from build123d import *

# Parameters (mm, degrees)
F1_DEPTH = 25.4
F2_R     = 3.175
F3_W     = 25.4
F3_H     = 6.35
F4_DEPTH = 53.976


with BuildPart() as f1:
    # F0 (on Front) → F1 (new body)
    with BuildSketch(Plane.XZ):
        with BuildLine():
            Line((-85.615239, 25.710709), (-159.144036, 1.439067))
            ThreePointArc((-159.144036, 1.439067), (-162.299532, -0.870485), (-163.503562, -4.590901))
            Line((-163.503562, -4.590901), (-163.503562, -26.984162))
            Line((-163.503562, -26.984162), (-81.740962, -26.984162))
            ThreePointArc((-81.740962, -26.984162), (-79.88109, -22.494034), (-75.390962, -20.634162))
            Line((-75.390962, -20.634162), (0, -20.634162))
            Line((0, -20.634162), (75.390962, -20.634162))
            ThreePointArc((75.390962, -20.634162), (79.88109, -22.494034), (81.740962, -26.984162))
            Line((81.740962, -26.984162), (163.503562, -26.984162))
            Line((163.503562, -26.984162), (163.503562, -4.590901))
            ThreePointArc((163.503562, -4.590901), (162.299532, -0.870485), (159.144036, 1.439067))
            Line((159.144036, 1.439067), (85.615239, 25.710709))
            ThreePointArc((85.615239, 25.710709), (81.685416, 26.668764), (77.65334, 26.990838))
            Line((77.65334, 26.990838), (0, 26.990838))
            Line((0, 26.990838), (-77.65334, 26.990838))
            ThreePointArc((-77.65334, 26.990838), (-81.685416, 26.668764), (-85.615239, 25.710709))
        make_face()
    extrude(amount=F1_DEPTH)

    # F2
    f2_edges = [f1.edges().sort_by_distance(p)[0] for p in [
        (-163.503562, -25.4, -15.787532),
        (-162.299532, -25.4, -0.870485),
        (-122.379638, -25.4, 13.574888),
        (122.379638, 0, 13.574888),
        (-163.503562, -12.7, -26.984162),
        (163.503562, -12.7, -26.984162),
    ]]
    fillet(f2_edges, radius=F2_R)

    # F3 (on face) → F4 (cut, through all)
    with BuildSketch(Plane.XY.offset(26.990838)):
        with Locations((0, -12.7)):
            Rectangle(F3_W, F3_H)
    extrude(amount=-F4_DEPTH, mode=Mode.SUBTRACT)


solid = f1.part
Design review of the part built by this model. Coordinates are the model's own, in mm. A direction names the side the tool comes from. Coordinates: 2 decimals unless noted, no trailing zeros. Order: outer loops, then holes, each group sorted by start corner. A loop starts at its lowest first (then second) coordinate and runs counter-clockwise, first axis right, second up.
Item 1: Take a section at B-B, the plane y = -12.75. Write out the cut boundary in (x, z) (3 decimals), then the cut area to 3 significant figures.
Item 2: For line 1 (Y direction, x = -2, z = -1) (3 decimals); line 2 (X direction, y = -13.5, z = -8); line 3 (Z direction, x = 10.5, y = -6.75), list the stretches that pass through material, from the lowest coordinate up.
Item 3: For pin 1 Ø12.5 at (x, y) = (0.5, -7) entering from -Z; pin 2 Ø8 at (x, y) = (111.5, -13) entering from +Z, all flat-tipped, find the tip position at first contact; note any pin that passes through.
Item 4: Take a section at C-C, the plane x = 20. Write out the cut boundary in (y, z) (3 decimals).
Item 5: Take a section at A-A, the plane z = -15. Write out the cut boundary in (x, y) (3 decimals).
Item 6: For faces 5 (the cylindrical face through (-81.629, -12.567, 26.678)), 6 (the flat face through (-1, -18, -20.634)), list the 3-axis set-ups (+Z, -Z, +X, -X, +Y, -Y) from which the entire face can be reached by the end or side of a thin tool; tool diameter is ignored.
Item 7: The part is to be moulded in two halves that separate along X. For faces 1 (the flat face through (1, -8, 26.991)), 2 (the flat face through (0, -9.525, 4)), 3 (the flat face through (-12.7, -13, 4)), 4 (the cylindrical face through (-162.27, -12.57, -0.83)), say which applies: pulls with the +X half, pulls with the -X half, needs draft (parallel to the pull), parting line crosses it, or undercut.
The answers:
1. outline: (-163.504, -23.809) arc R3.175 ccw to (-160.329, -26.984) - (-81.741, -26.984) arc R6.35 cw to (-75.391, -20.634) - (-12.7, -20.634) - (-12.7, 26.991) - (-77.653, 26.991) arc R25.4 ccw to (-85.615, 25.711) - (-159.144, 1.439) arc R6.35 ccw to (-163.504, -4.591) - close; (12.7, -20.634) - (75.391, -20.634) arc R6.35 cw to (81.741, -26.984) - (160.329, -26.984) arc R3.175 ccw to (163.504, -23.809) - (163.504, -4.591) arc R6.35 ccw to (159.144, 1.439) - (85.615, 25.711) arc R25.4 ccw to (77.653, 26.991) - (12.7, 26.991) - close
1. area: 13,200 mm2
2. line 1: y = -25.4 to -15.875, -9.525 to 0
2. line 2: x = -163.5 to -12.7, 12.7 to 163.5
2. line 3: z = -20.63 to 26.99
3. pin 1: stops at z = -20.63
3. pin 2: stops at z = 18.49
4. outline: (-25.4, -20.634) - (0, -20.634) - (0, 23.816) arc R3.175 ccw to (-3.175, 26.991) - (-22.225, 26.991) arc R3.175 ccw to (-25.4, 23.816) - close
5. outline: (-163.504, -22.225) arc R3.175 ccw to (-160.329, -25.4) - (160.329, -25.4) arc R3.175 ccw to (163.504, -22.225) - (163.504, -3.175) arc R3.175 ccw to (160.329, 0) - (-160.329, 0) arc R3.175 ccw to (-163.504, -3.175) - close; hole (-12.7, -15.875) - (12.7, -15.875) - (12.7, -9.525) - (-12.7, -9.525) - close
6. face 5: +Z, -X, +Y, -Y
6. face 6: -Z, +Y, -Y
7. face 1: needs draft
7. face 2: undercut
7. face 3: undercut
7. face 4: pulls with the -X half
